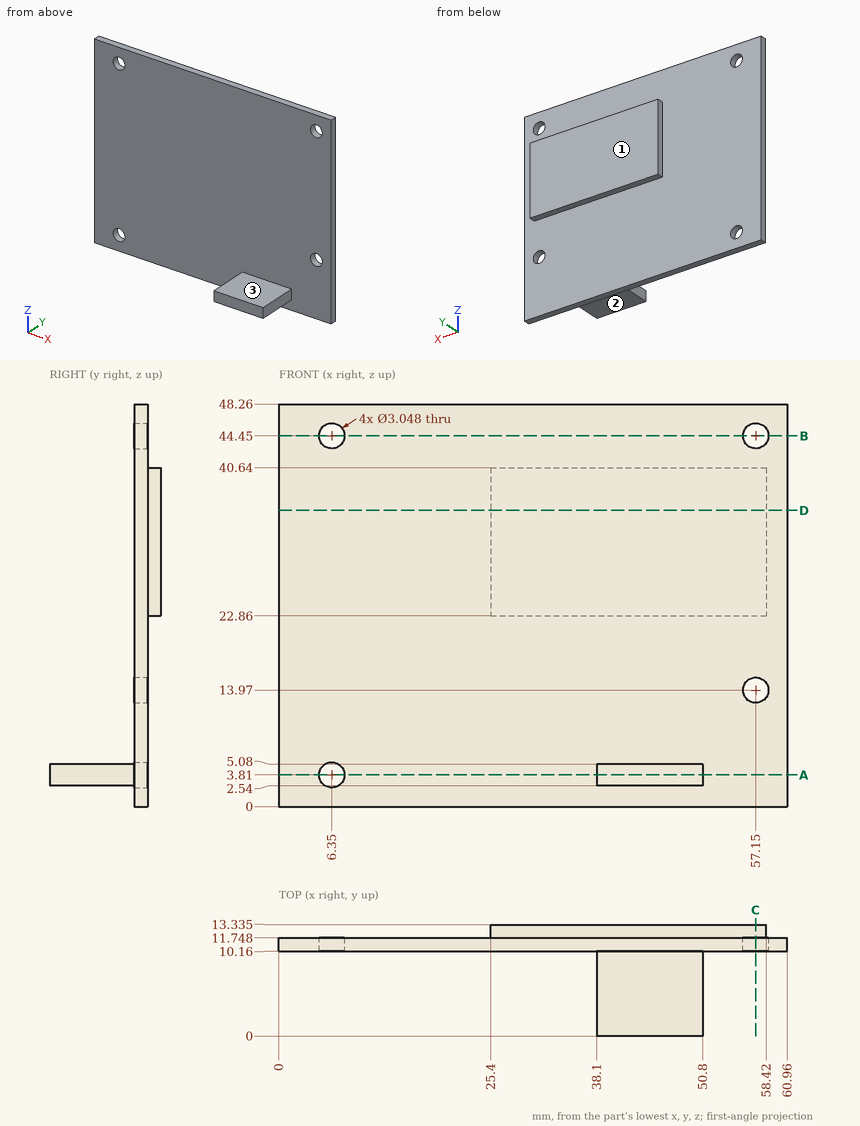
Source: three-view drawing plus pictorial views. Frame: mm from the lowest corner of the part. A direction names the side the tool comes from. Coordinates: 2 decimals unless noted, no trailing zeros. Loops run counter-clockwise (first coordinate to the right, second up) from the corner with the lowest first, then second, coordinate; pieces in that order, holes last. Notation, with made-up numbers: (61.5, 88) -> (97.5, 88) arc R16 cw to (97.5, 119) -> close; hole circle Ø11 at (-3.5, 56). An arc over 180 degrees is marked (long way). One line per item, written item: value.
(1) Pin query (flat end, axial travel): pin 1 Ø14.5 at (x, z) = (16, 34.5) entering from +Y; pin 2 Ø1.3 at (y, z) = (12.5, 35) entering from -X; pin 3 Ø2 at (y, z) = (5, 4.5) entering from -X. Return the tip coordinate at first contact, or that it passes through.
Answer below:
pin 1: stops at y = 11.75
pin 2: stops at x = 25.4
pin 3: stops at x = 38.1
(2) Cut plane D-D (z = 35.5). Output: boundary loops of the cut face in (x, y) (1 decimal).
Answer below:
outline: (0, 10.2) -> (61, 10.2) -> (61, 11.7) -> (58.4, 11.7) -> (58.4, 13.3) -> (25.4, 13.3) -> (25.4, 11.7) -> (0, 11.7) -> close
(3) Ray query, line 1 along X through (y, z) = (11.1, 44.45) (1 decimal); line 2 along Z through (x, y) = (57.15, 11.1) (1 decimal); line 3 along Z through (x, y) = (6.35, 11.45) (1 decimal). Return the intervals inside material, ascending.
Answer below:
line 1: x = 0 to 4.8, 7.9 to 55.6, 58.7 to 61
line 2: z = 0 to 12.4, 15.5 to 42.9, 46 to 48.3
line 3: z = 0 to 2.3, 5.3 to 42.9, 46 to 48.3
(4) Cut plane B-B (z = 44.45). Output: boundary loops of the cut face in (x, y) (1 decimal).
Answer below:
outline: (0, 10.2) -> (4.8, 10.2) -> (4.8, 11.7) -> (0, 11.7) -> close; (7.9, 10.2) -> (55.6, 10.2) -> (55.6, 11.7) -> (7.9, 11.7) -> close; (58.7, 10.2) -> (61, 10.2) -> (61, 11.7) -> (58.7, 11.7) -> close
(5) Cut plane A-A (z = 3.81). Output: boundary loops of the cut face in (x, y) (1 decimal).
Answer below:
outline: (0, 10.2) -> (4.8, 10.2) -> (4.8, 11.7) -> (0, 11.7) -> close; (7.9, 10.2) -> (38.1, 10.2) -> (38.1, 0) -> (50.8, 0) -> (50.8, 10.2) -> (61, 10.2) -> (61, 11.7) -> (7.9, 11.7) -> close
(6) Set-up query: the marked faces 1, 2 and 3. Return all of +Z, -Z, +X, -X, +Y, -Y with unobstructed straight access to the full face (end or side cutting, diameter ignored); none if empty.
Answer below:
face 1: +Z, -Z, +X, -X, +Y
face 2: -Z, +X, -X, -Y
face 3: +Z, +X, -X, -Y
(7) Cut plane C-C (x = 57.15). Output: boundary loops of the cut face in (y, z) (1 decimal).
Answer below:
outline: (10.2, 0) -> (11.7, 0) -> (11.7, 12.4) -> (10.2, 12.4) -> close; (10.2, 15.5) -> (11.7, 15.5) -> (11.7, 22.9) -> (13.3, 22.9) -> (13.3, 40.6) -> (11.7, 40.6) -> (11.7, 42.9) -> (10.2, 42.9) -> close; (10.2, 46) -> (11.7, 46) -> (11.7, 48.3) -> (10.2, 48.3) -> close
